```python
from build123d import *

# Parameters (mm, degrees)
SKETCH_1_R          = 34
EXTRUDE_1_DEPTH     = 4
SKETCH_2_R          = 30
SKETCH_2_R_2        = 26
EXTRUDE_2_DEPTH     = 8
SKETCH_3_R          = 2.5
SKETCH_3_R_2        = 1.5
CUT_EXTRUDE_1_DEPTH = 13
SKETCH_4_R          = 6
SKETCH_4_R_2        = 2.5
EXTRUDE_3_DEPTH     = 1
CHAMFER_1_SIZE      = 2
EXTRUDE_4_DEPTH     = 1


with BuildPart() as part:
    # 草图1 → 凸台-拉伸1 (new body)
    with BuildSketch(Plane(origin=(0, 0, 0), x_dir=(1, 0, 0), z_dir=(0, 1, 0))):
        Circle(SKETCH_1_R)
    extrude(amount=EXTRUDE_1_DEPTH)

    # 草图2 → 凸台-拉伸2 (add)
    with BuildSketch(Plane(origin=(0, 4, 0), x_dir=(1, 0, 0), z_dir=(0, 1, 0))):
        Circle(SKETCH_2_R)
        Circle(SKETCH_2_R_2, mode=Mode.SUBTRACT)
    extrude(amount=EXTRUDE_2_DEPTH)

    # 草图3 → 切除-拉伸1 (cut, through all)
    with BuildSketch(Plane.XZ):
        Circle(SKETCH_3_R)
        with Locations((0, 15)):
            Circle(SKETCH_3_R_2)
        with Locations((0, 22)):
            Circle(SKETCH_3_R_2)
        with Locations((15, 0)):
            Circle(SKETCH_3_R_2)
        with Locations((22, 0)):
            Circle(SKETCH_3_R_2)
        with Locations((0, -15)):
            Circle(SKETCH_3_R_2)
        with Locations((0, -22)):
            Circle(SKETCH_3_R_2)
        with Locations((-15, 0)):
            Circle(SKETCH_3_R_2)
        with Locations((-22, 0)):
            Circle(SKETCH_3_R_2)
    extrude(amount=-CUT_EXTRUDE_1_DEPTH, mode=Mode.SUBTRACT)

    # 草图4 → 凸台-拉伸3 (add)
    with BuildSketch(Plane.XZ):
        Circle(SKETCH_4_R)
        Circle(SKETCH_4_R_2, mode=Mode.SUBTRACT)
    extrude(amount=EXTRUDE_3_DEPTH)

    # 倒角1
    chamfer_1_edges = [part.edges().sort_by_distance(p)[0] for p in [
        (-34, 0, 0),
    ]]
    chamfer(chamfer_1_edges, length=CHAMFER_1_SIZE)

    # 草图5 → 凸台-拉伸4 (add)
    with BuildSketch(Plane.XZ):
        with BuildLine():
            Line((-19.445436483, -18.03122292), (-17.324116139, -15.909902577))
            ThreePointArc((-17.324116139, -15.909902577), (-15.909902577, -15.909902577), (-15.909902577, -17.324116139))
            Line((-15.909902577, -17.324116139), (-18.03122292, -19.445436483))
            ThreePointArc((-18.03122292, -19.445436483), (-19.445436483, -19.445436483), (-19.445436483, -18.03122292))
        make_face()
        with BuildLine():
            Line((-13.081475452, -20.152543264), (-15.202795796, -22.273863607))
            ThreePointArc((-15.202795796, -22.273863607), (-16.617009358, -22.273863607), (-16.617009358, -20.859650045))
            Line((-16.617009358, -20.859650045), (-14.495689014, -18.738329701))
            ThreePointArc((-14.495689014, -18.738329701), (-13.081475452, -18.738329701), (-13.081475452, -20.152543264))
        make_face()
        with BuildLine():
            Line((-20.152543264, -13.081475452), (-22.273863607, -15.202795796))
            ThreePointArc((-22.273863607, -15.202795796), (-22.273863607, -16.617009358), (-20.859650045, -16.617009358))
            Line((-20.859650045, -16.617009358), (-18.738329701, -14.495689014))
            ThreePointArc((-18.738329701, -14.495689014), (-18.738329701, -13.081475452), (-20.152543264, -13.081475452))
        make_face()
    extrude(amount=EXTRUDE_4_DEPTH)


solid = part.part
```
Verification items for the finished model (mm, model axes). A direction names the side the tool comes from. Round coordinates to 2 decimals unless told otherwise and drop trailing zeros. Answer as a JSON object with one key per item and string values. Group by question number.
Q1. Tool access check on faces 5 (the flat face through (-15.57, -0.49, -19.81)), 6 (the flat face through (-21.2, -0.49, -14.13)), 7 (the cylindrical face through (-29.97, 7.94, -1.32)). Record the directions out of +Z, -Z, +X, -X, +Y, -Y that give a thin tool (end or side, any length) a straight path to the whole face; none if there is none.
Q2. Mould release check, pull along X, two halves, no side actions. Record for faces 1 (the flat face through (5, 4, 0)), 2 (the cylindrical face through (-20.633, 7.944, 15.821)), 3 (the cylindrical face through (18.28, 2.99, -28.67)), 4 (the flat face through (-14.13, -0.49, -21.2)): released by +X, released by -X, zero draft, split by the parting line, or undercut.
Q3. Go/stop test with flat-tipped pins: pin 1 Ø6 at (x, y) = (12, 3.5) entering from -Z; pin 2 Ø4 at (x, y) = (0.5, 8) entering from +Z; pin 3 Ø4 at (x, y) = (-25, 5) entering from +Z. Record where each tip stops, or that it passes through.
Q4. Section check A-A, the plane y = 1. Give the number of separate pieces and of enclosed holes in the cut face, plus the area to 3 significant figures.
Q5. Thickness scan on line 1 (Z direction, x = 0, y = -0.45); line 2 (Y direction, x = 29.5, z = -10); line 3 (X direction, y = 8.25, z = 9). Record the ranges inside material, lowest first.
Found:
{
 "1": {"face 5": "-Y", "face 6": "+Z, -X, -Y", "face 7": "+Y"},
 "2": {"face 1": "undercut", "face 2": "undercut", "face 3": "split by the parting line", "face 4": "released by +X"},
 "3": {"pin 1": "stops at z = -32.79", "pin 2": "stops at z = 30", "pin 3": "stops at z = 24.79"},
 "4": {"separate pieces": "1", "enclosed holes": "9", "area": "3,350 mm^2"},
 "5": {"line 1": "z = -6 to -2.5, 2.5 to 6", "line 2": "y = 0 to 4", "line 3": "x = -28.62 to -24.39, 24.39 to 28.62"}
}
